from build123d import *

# Parameters (mm, degrees)
BOSS_EXTRUDE1_START = 5
SKETCH1_W           = 50
SKETCH1_H           = 50
BOSS_EXTRUDE1_DEPTH = 500
BOSS_EXTRUDE2_DEPTH = 110
BOSS_EXTRUDE3_DEPTH = 110
BOSS_EXTRUDE5_START = 110
BOSS_EXTRUDE5_DEPTH = 160
SKETCH1_3_W         = 240
SKETCH1_3_H         = 101.6
SKETCH1_3_W_2       = 50
SKETCH1_3_H_2       = 50
BOSS_EXTRUDE6_DEPTH = 6


with BuildPart() as part:
    # Sketch1 → Boss-Extrude1 (new body)
    with BuildSketch(Plane.XY.offset(40212.600196057).offset(BOSS_EXTRUDE1_START)):
        with Locations((-21671.561141737, -1732.035725356)):
            Rectangle(SKETCH1_W, SKETCH1_H)
    extrude(amount=BOSS_EXTRUDE1_DEPTH)

    # Sketch2 → Boss-Extrude2 (add)
    with BuildSketch(Plane(origin=(-21646.561141737, 0, 0), x_dir=(0, 0, -1), z_dir=(1, 0, 0))):
        Polygon((-40467.600196057, -1707.035725356), (-40467.600196057, -1757.035725356), (-40462.600196057, -1757.035725356), (-40462.600196057, -1712.035725356), (-40417.600196057, -1712.035725356), (-40417.600196057, -1707.035725356), align=None)
    extrude(amount=BOSS_EXTRUDE2_DEPTH)

    # Sketch3 → Boss-Extrude3 (add)
    with BuildSketch(Plane.ZY.offset(21696.561141737)):
        Polygon((40667.600196057, -1707.035725356), (40617.600196057, -1707.035725356), (40617.600196057, -1712.035725356), (40662.600196057, -1712.035725356), (40662.600196057, -1757.035725356), (40667.600196057, -1757.035725356), align=None)
        Polygon((40467.600196057, -1757.035725356), (40467.600196057, -1707.035725356), (40417.600196057, -1707.035725356), (40417.600196057, -1712.035725356), (40462.600196057, -1712.035725356), (40462.600196057, -1757.035725356), align=None)
        Polygon((40267.600196057, -1757.035725356), (40267.600196057, -1707.035725356), (40217.600196057, -1707.035725356), (40217.600196057, -1712.035725356), (40262.600196057, -1712.035725356), (40262.600196057, -1757.035725356), align=None)
    extrude(amount=BOSS_EXTRUDE3_DEPTH)

    # Sketch3<3> → Boss-Extrude5 (add)
    with BuildSketch(Plane.ZY.offset(21696.561141737).offset(BOSS_EXTRUDE5_START)):
        Polygon((40467.600196057, -1757.035725356), (40467.600196057, -1707.035725356), (40417.600196057, -1707.035725356), (40417.600196057, -1712.035725356), (40462.600196057, -1712.035725356), (40462.600196057, -1757.035725356), align=None)
    extrude(amount=BOSS_EXTRUDE5_DEPTH)

    # Sketch1<3> → Boss-Extrude6 (add)
    with BuildSketch(Plane.XY.offset(40212.600196057)):
        with Locations((-21670.561141737, -1731.342871453)):
            Rectangle(SKETCH1_3_W, SKETCH1_3_H)
        with Locations((-21671.561141737, -1732.035725356)):
            Rectangle(SKETCH1_3_W_2, SKETCH1_3_H_2, mode=Mode.SUBTRACT)
    extrude(amount=BOSS_EXTRUDE6_DEPTH)


solid = part.part
Geometry check sheet. Reference: the model listing, model coordinates, mm. A direction names the side the tool comes from. Give positions to 0.01 mm unless a question says otherwise; leave off trailing zeros. Write each loop counter-clockwise with the first axis right and the second up, starting at its lowest first coordinate (ties: lowest second). Pieces come first, ordered by that corner, then holes. Notation, with made-up numbers: M -6.75,49 L 0.25,49 A26 ccw 0.25,64 Z; hole C -37,-36 d8. An arc over 180 degrees is marked long. One line per question, with ' | ' between items.
1. Gauge pin test, flat ends, axial feed: pin 1 (3 mm diameter, centred on x = -21692.5, y = -1719.5, fed in from -Z); pin 2 (1 mm diameter, centred on y = -1719, z = 40297.5, fed in from +X); pin 3 (2 mm diameter, centred on y = -1726, z = 40497, fed in from -X). Record the tip position at first contact, or that the pin passes through.
Ans:
pin 1: z = 40217.6 | pin 2: x = -21646.56 | pin 3: x = -21696.56
2. Cross-section at A-A (x = -21589.5). Enter the section's corners in (y, z), plus the area to 3 significant figures.
Ans:
outline: M -1782.14,40212.6 L -1680.54,40212.6 L -1680.54,40218.6 L -1782.14,40218.6 Z; M -1757.04,40462.6 L -1712.04,40462.6 L -1712.04,40417.6 L -1707.04,40417.6 L -1707.04,40467.6 L -1757.04,40467.6 Z | area: 1,080 mm2
3. Cross-section at B-B (x = -21744.5). Enter the section's corners in (y, z).
Ans:
outline: M -1782.14,40212.6 L -1680.54,40212.6 L -1680.54,40218.6 L -1707.04,40218.6 L -1707.04,40267.6 L -1757.04,40267.6 L -1757.04,40262.6 L -1712.04,40262.6 L -1712.04,40218.6 L -1782.14,40218.6 Z; M -1757.04,40462.6 L -1712.04,40462.6 L -1712.04,40417.6 L -1707.04,40417.6 L -1707.04,40467.6 L -1757.04,40467.6 Z; M -1757.04,40662.6 L -1712.04,40662.6 L -1712.04,40617.6 L -1707.04,40617.6 L -1707.04,40667.6 L -1757.04,40667.6 Z
4. Mould release check, pull along X, two halves, no side actions. Record for faces 5 (the face through (-21751, -1734, 40662.6)), 6 (the face through (-21671, -1732, 40217.6)), 7 (the face through (-21536.561, -1721, 40463)): released by +X, released by -X, zero draft, split by the parting line, or undercut.
Ans:
face 5: zero draft | face 6: undercut | face 7: released by +X
5. Scan lines: line 1 along Z through (x, y) = (-21788, -1707.5); line 2 along Z through (x, y) = (-21633.5, -1748); line 3 along Z through (x, y) = (-21754, -1755). Record each from-to range of solid material in increasing order. Write a range as from..to.
Ans:
line 1: 40212.6..40267.6, 40417.6..40467.6, 40617.6..40667.6 | line 2: 40212.6..40218.6, 40462.6..40467.6 | line 3: 40212.6..40218.6, 40262.6..40267.6, 40462.6..40467.6, 40662.6..40667.6
6. Cross-section at C-C (y = -1744.5). Enter the section's corners in (x, z).
Ans:
outline: M -21966.56,40462.6 L -21696.56,40462.6 L -21696.56,40267.6 L -21806.56,40267.6 L -21806.56,40262.6 L -21696.56,40262.6 L -21696.56,40218.6 L -21790.56,40218.6 L -21790.56,40212.6 L -21696.56,40212.6 L -21696.56,40217.6 L -21646.56,40217.6 L -21646.56,40212.6 L -21550.56,40212.6 L -21550.56,40218.6 L -21646.56,40218.6 L -21646.56,40462.6 L -21536.56,40462.6 L -21536.56,40467.6 L -21646.56,40467.6 L -21646.56,40717.6 L -21696.56,40717.6 L -21696.56,40667.6 L -21806.56,40667.6 L -21806.56,40662.6 L -21696.56,40662.6 L -21696.56,40467.6 L -21966.56,40467.6 Z
7. Cross-section at D-D (z = 40433). Enter the section's corners in (x, y).
Ans:
outline: M -21966.56,-1712.04 L -21696.56,-1712.04 L -21696.56,-1757.04 L -21646.56,-1757.04 L -21646.56,-1712.04 L -21536.56,-1712.04 L -21536.56,-1707.04 L -21966.56,-1707.04 Z
8. Set-up check for faces 1 (the face through (-21592, -1732, 40467.6)), 2 (the face through (-21646, -1731, 40218.6)), 3 (the face through (-21751, -1732, 40267.6)), 4 (the face through (-21751, -1712.036, 40640)): record each of +Z, -Z, +X, -X, +Y, -Y from which the full face is reachable in a straight line by a thin tool's end or side.
Ans:
face 1: +Z, +X, +Y, -Y | face 2: none | face 3: -X, +Y, -Y | face 4: -X, -Y
